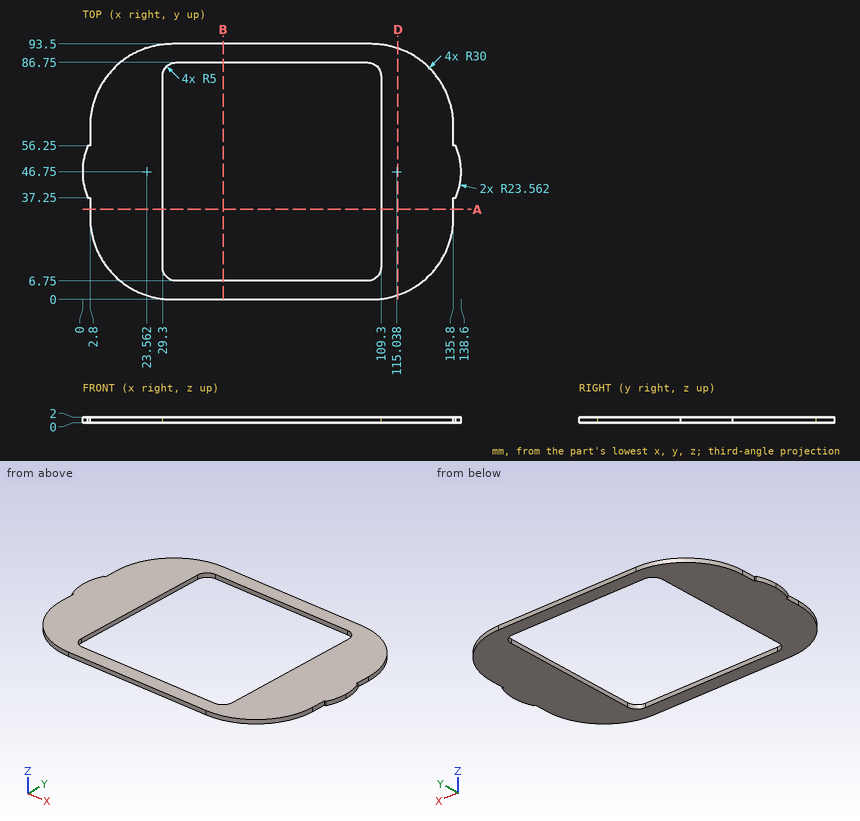
Print and shaded views of the part. All mm, measured from the part's lowest x, y and z. Coordinates: 2 decimals unless noted, no trailing zeros. Loops run counter-clockwise (first coordinate to the right, second up) from the corner with the lowest first, then second, coordinate; pieces in that order, holes last. Notation, with made-up numbers: M 87,-40 L 137,-40 A22 cw 137,-28 Z; hole C 31.25,-15.75 d8. An arc over 180 degrees is marked long. Use a Markdown table: item, result. Add a question column.
Q1. Probe L1, parallel to X at y = 29, z = 0.75; L2, parallel to Y at x = 82, z = 1.05; L3, parallel to X at y = 44.5, z = 1.8. List the from-to ranges inside material, lowest first.
Q2. Pin check, flat tips, straight feed: P1, Ø0.6, axis at x = 136.5, z = 0.5, coming from the -Y side; P2, Ø4, axis at x = 108.5, y = 62.5, coming from the +Z side; P3, Ø0.6, axis at y = 56, z = 1, coming from the -X side (1 decimal); P4, Ø1, axis at y = 32.5, z = 1, coming from the +X side. Stop position of each tip, or through.
Q3. Cut at D-D (x = 115.5). Write the cut outline in (y, z).
Q4. Cut at B-B (x = 51.5). Write the cut outline in (y, z), and give its area (3 significant figures).
Q5. Cut at A-A (y = 33). Write the cut outline in (x, z), and give its area (3 significant figures).
Worked out:
| question | item | result |
|---|---|---|
| 1 | L1 | x = 2.82 to 29.3, 109.3 to 135.78 |
| 1 | L2 | y = 0 to 6.75, 86.75 to 93.5 |
| 1 | L3 | x = 0.11 to 29.3, 109.3 to 138.49 |
| 2 | P1 | stops at y = 37.25 |
| 2 | P2 | stops at z = 2 |
| 2 | P3 | stops at x = 1.8 |
| 2 | P4 | stops at x = 135.8 |
| 3 | outline | M 1.61,0 L 91.89,0 L 91.89,2 L 1.61,2 Z |
| 4 | outline | M 0,0 L 6.75,0 L 6.75,2 L 0,2 Z; M 86.75,0 L 93.5,0 L 93.5,2 L 86.75,2 Z |
| 4 | area | 27.0 mm2 |
| 5 | outline | M 2.8,0 L 29.3,0 L 29.3,2 L 2.8,2 Z; M 109.3,0 L 135.8,0 L 135.8,2 L 109.3,2 Z |
| 5 | area | 106 mm2 |
